Part model, mm, in its own coordinate system. A direction names the side the tool comes from. Give positions to 0.01 mm unless a question says otherwise; leave off trailing zeros. Write each loop counter-clockwise with the first axis right and the second up, starting at its lowest first coordinate (ties: lowest second). Pieces come first, ordered by that corner, then holes.
```python
from build123d import *

# Parameters (mm, degrees)
SKETCH1_W           = 76.2
SKETCH1_H           = 203.2
BOSS_EXTRUDE1_DEPTH = 4.3434
SKETCH2_W           = 12.7
SKETCH2_H           = 6.35
BOSS_EXTRUDE2_DEPTH = 4.3434
SKETCH3_W           = 12.0904
SKETCH3_H           = 19.05
CUT_EXTRUDE1_DEPTH  = 112.571841199


with BuildPart() as part:
    # Sketch1 → Boss-Extrude1 (new body)
    with BuildSketch(Plane.XY):
        Rectangle(SKETCH1_W, SKETCH1_H)
    extrude(amount=BOSS_EXTRUDE1_DEPTH)

    # Sketch2 → Boss-Extrude2 (add)
    with BuildSketch(Plane.XY.offset(4.3434)):
        with Locations((0, 101.6)):
            Rectangle(SKETCH2_W, SKETCH2_H)
        with Locations((-25.4, 101.6)):
            Rectangle(SKETCH2_W, SKETCH2_H)
        with Locations((25.4, 101.6)):
            Rectangle(SKETCH2_W, SKETCH2_H)
        with Locations((25.4, -101.6)):
            Rectangle(SKETCH2_W, SKETCH2_H)
        with Locations((-25.4, -101.6)):
            Rectangle(SKETCH2_W, SKETCH2_H)
        with Locations((0, -101.6)):
            Rectangle(SKETCH2_W, SKETCH2_H)
    extrude(amount=-BOSS_EXTRUDE2_DEPTH)

    # Sketch3 → Cut-Extrude1 (cut, through all)
    with BuildSketch(Plane.XY.offset(4.3434)):
        with Locations((38.1, 0)):
            Rectangle(SKETCH3_W, SKETCH3_H)
        with Locations((38.1, 35.052)):
            Rectangle(SKETCH3_W, SKETCH3_H)
        with Locations((38.1, 70.104)):
            Rectangle(SKETCH3_W, SKETCH3_H)
        with Locations((38.1, -70.104)):
            Rectangle(SKETCH3_W, SKETCH3_H)
        with Locations((38.1, -35.052)):
            Rectangle(SKETCH3_W, SKETCH3_H)
        with Locations((-38.1, -35.052)):
            Rectangle(SKETCH3_W, SKETCH3_H)
        with Locations((-38.1, -70.104)):
            Rectangle(SKETCH3_W, SKETCH3_H)
        with Locations((-38.1, 70.104)):
            Rectangle(SKETCH3_W, SKETCH3_H)
        with Locations((-38.1, 35.052)):
            Rectangle(SKETCH3_W, SKETCH3_H)
        with Locations((-38.1, 0)):
            Rectangle(SKETCH3_W, SKETCH3_H)
    extrude(amount=-CUT_EXTRUDE1_DEPTH, mode=Mode.SUBTRACT)


solid = part.part
```
1) Wall check: L1, parallel to Y at x = 10.5, z = 2.15; L2, parallel to X at y = -74, z = 0.3. Give the ranges that are in metal, low to high.
Answers follow:
L1: y = -101.6 to 101.6
L2: x = -32.05 to 32.05
2) Two-plate mould, pull along X, no slides. Class faces 1 (the face through (35, -60.579, 2)), 2 (the face through (-13, -101.6, 2)), 3 (the face through (38.1, 17, 2)): +X half, -X half, draft (parallel to the pull), parting line (faces both ways), or undercut.
Answers follow:
face 1: draft
face 2: undercut
face 3: +X half
3) Pin check, flat tips, straight feed: pin 1 Ø1.5 at (y, z) = (62.5, 2) entering from +X; pin 2 Ø2 at (x, z) = (-34.5, 3) entering from -Y; pin 3 Ø1.6 at (y, z) = (-103.5, 1.5) entering from +X. Stop position of each tip, or through.
Answers follow:
pin 1: stops at x = 32.05
pin 2: stops at y = -101.6
pin 3: stops at x = 31.75
4) Saw through at B-B, the plane y = 3. Write the cut outline in (x, z).
Answers follow:
outline: (-32.05, 0) - (32.05, 0) - (32.05, 4.34) - (-32.05, 4.34) - close
5) 3-axis set-ups, long thin cutter, end or side, ignore diameter. For faces 4 (the face through (-32.055, -35, 2)), 5 (the face through (35, -101.6, 2)), 6 (the face through (35, -44.577, 2)): which of +Z, -Z, +X, -X, +Y, -Y reach the whole face in a straight line?
Answers follow:
face 4: +Z, -Z, -X
face 5: +Z, -Z, +X, -Y
face 6: +Z, -Z, +X
6) Saw through at A-A, the plane x = -8.5. Write the cut outline in (y, z).
Answers follow:
outline: (-101.6, 0) - (101.6, 0) - (101.6, 4.34) - (-101.6, 4.34) - close
